```python
from build123d import *

# Parameters (mm, degrees)
F1_DEPTH = 57.15
F3_R     = 6.35
F4_DEPTH = 12.7
F6_R     = 6.3501577228
F7_DEPTH = 12.7


with BuildPart() as f1:
    # F0 (on Front) → F1 (new body)
    with BuildSketch(Plane.XZ):
        with BuildLine():
            Line((-836.8502492905, 108.3186204791), (-868.6002492905, 108.3186204791))
            Line((-868.6002492905, 108.3186204791), (-868.6002492905, 95.6186204791))
            Line((-868.6002492905, 95.6186204791), (-792.4002492905, 95.6186204791))
            Line((-792.4002492905, 95.6186204791), (-716.2002492905, 95.6186204791))
            Line((-716.2002492905, 95.6186204791), (-716.2002492905, 108.3186204791))
            Line((-716.2002492905, 108.3186204791), (-747.9502492905, 108.3186204791))
            Line((-747.9502492905, 108.3186204791), (-747.9502492905, 140.0686204791))
            Line((-747.9502492905, 140.0686204791), (-760.6336884818, 140.0686204791))
            ThreePointArc((-760.6336884818, 140.0686204791), (-769.5781696434, 117.9718545123), (-791.3746345435, 108.3186204791))
            ThreePointArc((-791.3746345435, 108.3186204791), (-791.8873750687, 108.3062001425), (-792.4002492905, 108.3020596705))
            ThreePointArc((-792.4002492905, 108.3020596705), (-792.9131235123, 108.3062001425), (-793.4258640374, 108.3186204791))
            ThreePointArc((-793.4258640374, 108.3186204791), (-815.2223289375, 117.9718545123), (-824.1668100991, 140.0686204791))
            Line((-824.1668100991, 140.0686204791), (-836.8502492905, 140.0686204791))
            Line((-836.8502492905, 140.0686204791), (-836.8502492905, 108.3186204791))
        make_face()
    extrude(amount=F1_DEPTH)

    # F3 (on offset) → F4 (cut)
    with BuildSketch(Plane.XY.offset(108.3186204791)):
        with Locations((-852.1803617477, -27.7651418)):
            Circle(F3_R)
    extrude(amount=-F4_DEPTH, mode=Mode.SUBTRACT)

    # F6 (on offset) → F7 (cut)
    with BuildSketch(Plane.XY.offset(108.3186204791)):
        with Locations((-732.0292592049, -28.564395383)):
            Circle(F6_R)
    extrude(amount=-F7_DEPTH, mode=Mode.SUBTRACT)


solid = f1.part
```
Geometry: final body of the model. Coordinates: model frame, mm. A direction names the side the tool comes from. Round coordinates to 2 decimals unless told otherwise and drop trailing zeros. Write each loop counter-clockwise with the first axis right and the second up, starting at its lowest first coordinate (ties: lowest second). Pieces come first, ordered by that corner, then holes. Notation, with made-up numbers: M -17,31 L 3,31 A20 ccw 3,52 Z; hole C 59,67.5 d2. An arc over 180 degrees is marked long. Answer in a Markdown table with one row per item. Add a question column.
(1) Reachability of faces 1 (the face through (-793, -28, 95.619)), 2 (the face through (-732, -22, 108.319)), 3 (the face through (-853, -35, 108.319)) from +Z, -Z, +X, -X, +Y, -Y: full face, straight path, thin tool, end or side. Return the list, or none.
(2) Draft query along X for faces 4 (the face through (-793, 0, 108)), 5 (the face through (-747.95, -28, 124)), 6 (the face through (-725.97, -26.66, 102.06)). Return one class per face: pulls with the +X half, pulls with the -X half, needs draft (parallel to the pull), parting line crosses it, or undercut.
(3) Cut plane C-C, the plane x = -850. Return the cut outline in (y, z).
(4) Ray query, L1, parallel to X at y = -33, z = 107.5; L2, parallel to X at y = -24.5, z = 103; L3, parallel to Z at x = -861.5, y = -3.5. Return the intervals inside material, ascending.
(5) Cut plane D-D, the plane y = -25. Return the cut outline in (x, z).
(6) Contact query for flat-ended pins moving along their axis: pin 1 (6 mm diameter, centred on y = -30, z = 130.5, fed in from +X); pin 2 (9.5 mm diameter, centred on x = -857.5, y = -27, fed in from +Z); pin 3 (10 mm diameter, centred on x = -852.18, y = -27.77, fed in from +Z); pin 4 (16 mm diameter, centred on y = -24.5, z = 118, fed in from -X). Output: stop coordinate, or through.
(7) Cut plane A-A, the plane z = 110.5. Return the cut outline in (x, y), then the cut area to 3 significant figures.
(8) Cut plane B-B, the plane y = -14. Return the cut outline in (x, z).
Established:
| question | item | result |
|---|---|---|
| 1 | face 1 | -Z, +X, -X, +Y, -Y |
| 1 | face 2 | +Z, +X, +Y, -Y |
| 1 | face 3 | +Z, -X, +Y, -Y |
| 2 | face 4 | needs draft |
| 2 | face 5 | pulls with the +X half |
| 2 | face 6 | undercut |
| 3 | outline | M -57.15,95.62 L -33.73,95.62 L -33.73,108.32 L -57.15,108.32 Z; M -21.8,95.62 L 0,95.62 L 0,108.32 L -21.8,108.32 Z |
| 4 | L1 | -868.6 to -855.77, -848.59 to -736.57, -727.49 to -716.2 |
| 4 | L2 | -868.6 to -857.63, -846.73 to -736.91, -727.15 to -716.2 |
| 4 | L3 | 95.62 to 108.32 |
| 5 | outline | M -868.6,95.62 L -857.9,95.62 L -857.9,108.32 L -868.6,108.32 Z; M -846.46,95.62 L -737.28,95.62 L -737.28,108.32 L -747.95,108.32 L -747.95,140.07 L -760.63,140.07 A31.77 cw -824.17,140.07 L -836.85,140.07 L -836.85,108.32 L -846.46,108.32 Z; M -726.77,95.62 L -716.2,95.62 L -716.2,108.32 L -726.77,108.32 Z |
| 6 | pin 1 | x = -747.95 |
| 6 | pin 2 | z = 108.32 |
| 6 | pin 3 | through |
| 6 | pin 4 | x = -836.85 |
| 7 | outline | M -836.85,-57.15 L -804.01,-57.15 L -804.01,0 L -836.85,0 Z; M -780.79,-57.15 L -747.95,-57.15 L -747.95,0 L -780.79,0 Z |
| 7 | area | 3,750 mm² |
| 8 | outline | M -868.6,95.62 L -716.2,95.62 L -716.2,108.32 L -747.95,108.32 L -747.95,140.07 L -760.63,140.07 A31.77 cw -824.17,140.07 L -836.85,140.07 L -836.85,108.32 L -868.6,108.32 Z |
